The listing builds one solid part. Answer for the finished solid, in the listing's coordinates (mm). A direction names the side the tool comes from. Give positions to 0.01 mm unless a question says otherwise; leave off trailing zeros. Loops run counter-clockwise (first coordinate to the right, second up) from the corner with the lowest first, then second, coordinate; pieces in that order, holes last. Notation, with made-up numbers: M -39,71 L -30,71 A27 cw -30,87 Z; hole C 17,31.5 d11. An arc over 180 degrees is marked long. Return JSON: item names as keys, results as strings.
Autodesk Inventor part; units mm, degrees
ref_plane "Work Plane2" through (0, -10.6667, 0) normal (-1, 0, 0) x (0, 1, 0)
ref_plane "Work Plane4" through (0, 15.0859, -8.6603) normal (0, 0.8164966, 0.5773503) x (1, 0, 0)
ref_plane "YZ Plane" through (0, 0, 0) normal (1, 0, 0) x (0, 1, 0)
sketch "Sketch3" plane through (0, 0, 0) normal (0, 0, 1) x (1, 0, 0)
  line L0 (0, 27.3333) -> (-41, -13.6667)
  line L1 (-41, -13.6667) -> (41, -13.6667)
  line L2 (41, -13.6667) -> (0, 27.3333)
  line L3 (41, -13.6667) -> (-20.5, 6.8333) construction
  line L4 (-41, -13.6667) -> (20.5, 6.8333) construction
  point P0 (0, 0)
  dimension "d7" = 90
  dimension "d8" = 45
  dimension "d9" = 82
extrude "Extrusion1" add sketch "Sketch3" against normal blind 3 draft -45
sketch "Sketch4" plane through (0, 0, 0) normal (0, 0, 1) x (1, 0, 0)
  line L0 (-33.7574, -10.6667) -> (33.7574, -10.6667)
  line L1 (0, 23.0907) -> (-33.7574, -10.6667)
  point P0 (0, 0)
  point P1 (0, -10.6667)
ref_plane "Work Plane2" through (0, -10.6667, 0) normal (-1, 0, 0) x (0, 1, 0)
sketch "Sketch5" plane through (0, -10.6667, 0) normal (-1, 0, 0) x (0, 1, 0)
  line L0 (38, 0) -> (-3, 0) construction
  line L1 (-3, 0) -> (10.6667, 19.3276) construction
  line L2 (38, 0) -> (10.6667, 19.3276)
  line L3 (-3, 0) -> (38, 0)
  point P0 (10.6667, 0)
  dimension "d18" = 23.6714
pattern_circular "Circular Pattern1" count 3 over 360 about axis through (0, 27.3333, 0) along (0, -0.8164966, -0.5773503) of "Extrusion1"
sketch "Sketch6" plane through (0, -10.6667, 0) normal (-1, 0, 0) x (0, 1, 0)
  line L0 (38, 0) -> (-3, 0)
  line L1 (38, 0) -> (38, 57.9828)
  line L2 (38, 57.9828) -> (-3, 0)
  line L3 (38, 0) -> (-3, 0)
  line L4 (48.9333, -7.731) -> (-27.6, 46.3862)
  point P0 (10.6667, 0)
  point P1 (25.7526, 8.6603)
  dimension "d20" = 15
ref_plane "Work Plane4" through (0, 15.0859, -8.6603) normal (0, 0.8164966, 0.5773503) x (1, 0, 0)
ref_plane "Work Plane3" through (-41, -13.6667, 0) normal (0, 0.8164966, 0.5773503) x (1, 0, 0)
sketch "Sketch7" plane through (0, 15.0859, -8.6603) normal (0, 0.8164966, 0.5773503) x (1, 0, 0)
  line L0 (12.0072, -6.9324) -> (0, 13.8647)
  line L1 (0, 13.8647) -> (-12.0072, -6.9324)
  line L2 (-12.0072, -6.9324) -> (12.0072, -6.9324)
  line L3 (0, 21.2132) -> (18.3712, -10.6066)
  line L4 (18.3712, -10.6066) -> (-18.3712, -10.6066)
  line L5 (-18.3712, -10.6066) -> (0, 21.2132)
  line L6 (-12.0072, -6.9324) -> (0, 13.8647)
  line L7 (12.0072, -6.9324) -> (0, 13.8647)
  line L8 (12.0072, -6.9324) -> (-12.0072, -6.9324)
  point P0 (0, -15.7809)
extrude "Extrusion2" add sketch "Sketch7" along normal up to next contours L2 L1 L0
(1) Determine the mould class of faces 3 (the flat face through (-1, 3, 0)), 4 (the flat face through (12.81, 10.28, -20.45)), 5 (the flat face through (12.671, 14.662, -17.108)) for opening direction X: released by +X, released by -X, zero draft, split by the parting line, or undercut.
Values follow:
{"face 3": "zero draft", "face 4": "undercut", "face 5": "released by +X"}
(2) Given pin 1 (12 mm diameter, centred on x = 3, y = 5.5, fed in from -Z); pin 2 (12 mm diameter, centred on x = -25.5, z = -11.5, fed in from +Y); pin 3 (17.5 mm diameter, centred on x = -10.5, y = 3.5, fed in from -Z), each flat-ended and moving along its own axis, determine where each tip first touches the part or whether it passes through.
Values follow:
{"pin 1": "z = -3.59", "pin 2": "y = 7.83", "pin 3": "z = -35.53"}
(3) The part is cut by section D-D (z = -5). Determine the outline of the cut face in (x, y).
Values follow:
{"outline": "M -37.46,-10.13 L -32.34,-9.25 L -10.59,12.5 L 10.59,12.5 L 32.34,-9.25 L 37.46,-10.13 L 0,27.33 Z"}
(4) The part is cut by section A-A (z = -14). Determine the outline of the cut face in (x, y).
Values follow:
{"outline": "M -31.1,-3.77 L -25.98,-2.89 L -4.23,18.86 L 4.23,18.86 L 25.98,-2.89 L 31.1,-3.77 L 0,27.33 Z"}
(5) A tool of negligible diameter and unlimited length cuts with its end or side. For faces 1 (the flat face through (-12.097, 15.236, -17.92)), 2 (the flat face through (-18.428, 6.814, -28.351)), from which of +Z, -Z, +X, -X, +Y, -Y can it reach the whole face along a straight path? Write none if from no direction.
Values follow:
{"face 1": "+Z, -Z, -X, +Y", "face 2": "-Z, -Y"}
(6) The part is cut by section B-B (y = 2.5). Determine the outline of the cut face in (x, z), and give its area (3 significant figures).
Values follow:
{"outline": "M -24.83,-22.86 L -20.59,-21.62 L -20.59,-3 L 20.59,-3 L 20.59,-21.62 L 24.83,-22.86 L 24.83,0 L -24.83,0 Z", "area": "312 mm²"}
(7) The part is cut by section C-C (x = 17). Determine the outline of the cut face in (y, z).
Values follow:
{"outline": "M -13.67,0 L -10.67,-3 L 6.09,-3 L 6.09,-26.7 L 10.33,-33.94 L 10.33,0 Z"}
(8) Straight lines are drawn through the part: line 1 along X through (y, z) = (10.5, -21); line 2 along Z through (x, y) = (-0.5, 9); line 3 along X through (y, z) = (7, -6). For each, find the intervals that lie inside material, in ascending order.
Values follow:
{"line 1": "-16.83 to -12.59, 12.59 to 16.83", "line 2": "-3 to 0", "line 3": "-20.33 to -16.09, 16.09 to 20.33"}
